```python
from build123d import *

# Parameters (mm, degrees)
F1_DEPTH  = 426
F3_DEPTH  = 4
F4_R      = 2
F7_DEPTH  = 4
F10_DEPTH = 4


# Not quite as in the source:
# - a feature names something its author has since deleted; it is built from what else it names


with BuildPart() as f1:
    # F0 (on Top) → F1 (new body)
    with BuildSketch(Plane.XY):
        Polygon((-200, -343), (0, -343), (0, 0), (-495, 0), (-495, -1303), (-491, -1303), (-491, -4), (-4, -4), (-4, -339), (-204, -339), (-204, -1303), (-200, -1303), align=None)
    extrude(amount=F1_DEPTH)

    # F2 (on Top) → F3 (join)
    with BuildSketch(Plane.XY):
        Polygon((0, 0), (-495, 0), (-495, -1303), (-200, -1303), (-200, -343), (0, -343), align=None)
    extrude(amount=-F3_DEPTH)

    # F4
    f4_edges = [f1.edges().sort_by_distance(p)[0] for p in [
        (-200, -823, -4),
        (-495, -651.5, -4),
        (-247.5, 0, -4),
        (0, -343, 211),
        (0, 0, 211),
    ]]
    fillet(f4_edges, radius=F4_R)

    # F6 (on offset) → F7 (join)
    with BuildSketch(Plane.XZ.offset(1003)):
        Polygon((-491, 0), (-269, 0), (-491, 335), align=None)
    extrude(amount=F7_DEPTH)

    # F9 (on offset) → F10 (join)
    with BuildSketch(Plane.XZ.offset(403)):
        Polygon((-204, 335), (-426, 0), (-204, 0), align=None)
    extrude(amount=F10_DEPTH)


solid = f1.part
```
Verification items for the finished model (mm, model axes). A direction names the side the tool comes from. Round coordinates to 2 decimals unless told otherwise and drop trailing zeros. Write each loop counter-clockwise with the first axis right and the second up, starting at its lowest first coordinate (ties: lowest second). Pieces come first, ordered by that corner, then holes.
1. Gauge pin test, flat ends, axial feed: P1, Ø3, axis at x = -381, y = -708, coming from the +Z side; P2, Ø2, axis at x = -246, z = 211, coming from the -Y side; P3, Ø6, axis at y = -408, z = 178, coming from the +X side. Record the tip position at first contact, or that the pin passes through.
2. Section check D-D on y = -282. Enter the section's corners in (x, z), plus the area to 3 significant figures.
3. Section check B-B on x = -50. Enter the section's corners in (y, z), plus the area to 3 significant figures.
4. Scan lines: L1, parallel to Y at x = -372.5, z = 80; L2, parallel to X at y = -995, z = 228.5; L3, parallel to Y at x = -102, z = 125. Record each from-to range of solid material in increasing order.
5. Access from +Z, -Z, +X, -X, +Y, -Y to the whole of each face (thin tool, end or side, straight path). Record for faces 1 (the flat face through (-200, -830, 215)), 2 (the flat face through (-378.45, -1004.97, 165.16)), 3 (the flat face through (-495, -642, 215)), 4 (the flat face through (-431, -1003, 95)), 5 (the flat face through (-305, -499, -4)).
6. Draft check along X on faces 6 (the flat face through (0, -174, 214)), 7 (the flat face through (-245, 0, 215)), 8 (the flat face through (-491, -663, 210)). Enter one of: +X half, -X half, draft (parallel to the pull), parting line (faces both ways), or undercut.
7. Section check A-A on y = -830.5. Enter the section's corners in (x, z), plus the area to 3 significant figures.
8. Section check C-C on z = 78. Enter the section's corners in (x, y), plus the area to 3 significant figures.
Answer:
1. P1: stops at z = 0
1. P2: stops at y = -407
1. P3: stops at x = -200
2. outline: (-495, -2) arc R2 ccw to (-493, -4) - (0, -4) - (0, 426) - (-4, 426) - (-4, 0) - (-491, 0) - (-491, 426) - (-495, 426) - close
2. area: 5,390 mm2
3. outline: (-343, -4) - (-2, -4) arc R2 ccw to (0, -2) - (0, 426) - (-4, 426) - (-4, 0) - (-339, 0) - (-339, 426) - (-343, 426) - close
3. area: 4,780 mm2
4. L1: y = -1007 to -1003, -407 to -403, -4 to 0
4. L2: x = -495 to -491, -204 to -200
4. L3: y = -343 to -339, -4 to 0
5. face 1: +Z, -Z, +X, -Y
5. face 2: +Z, -Y
5. face 3: +Z, -Z, -X, +Y, -Y
5. face 4: +Z
5. face 5: -Z, +X, -X, +Y, -Y
6. face 6: +X half
6. face 7: draft
6. face 8: undercut
7. outline: (-495, -2) arc R2 ccw to (-493, -4) - (-202, -4) arc R2 ccw to (-200, -2) - (-200, 426) - (-204, 426) - (-204, 0) - (-491, 0) - (-491, 426) - (-495, 426) - close
7. area: 4,590 mm2
8. outline: (-495, -1303) - (-491, -1303) - (-491, -1007) - (-320.69, -1007) - (-320.69, -1003) - (-491, -1003) - (-491, -4) - (-4, -4) - (-4, -339) - (-204, -339) - (-204, -403) - (-374.31, -403) - (-374.31, -407) - (-204, -407) - (-204, -1303) - (-200, -1303) - (-200, -343) - (-2, -343) arc R2 ccw to (0, -341) - (0, -2) arc R2 ccw to (-2, 0) - (-495, 0) - close
8. area: 14,500 mm2
